from build123d import *

# Parameters (mm, degrees)
F0_W     = 35
F0_H     = 10.25
F0_W_2   = 10.25
F0_H_2   = 25
F1_DEPTH = 10
F2_R     = 10
F2_R_2   = 15
F3_DEPTH = 10


with BuildPart() as f1:
    # F0 (on Top) → F1 (new body)
    with BuildSketch(Plane.XY):
        with BuildLine():
            Line((140, 110), (-140, 110))
            ThreePointArc((-140, 110), (-147.071068, 107.071068), (-150, 100))
            Line((-150, 100), (-150, -100))
            ThreePointArc((-150, -100), (-147.071068, -107.071068), (-140, -110))
            Line((-140, -110), (140, -110))
            ThreePointArc((140, -110), (147.071068, -107.071068), (150, -100))
            Line((150, -100), (150, 100))
            ThreePointArc((150, 100), (147.071068, 107.071068), (140, 110))
        make_face()
        Polygon((-105.125, -100.125), (-140.125, -100.125), (-140.125, -75.125), (-129.875, -75.125), (-129.875, -89.878049), (-105.125, -89.875), align=None, mode=Mode.SUBTRACT)
        with Locations((-52.625, -95)):
            Rectangle(F0_W, F0_H, mode=Mode.SUBTRACT)
        with Locations((-135, -37.625)):
            Rectangle(F0_W_2, F0_H_2, mode=Mode.SUBTRACT)
        with Locations((52.625, -95)):
            Rectangle(F0_W, F0_H, mode=Mode.SUBTRACT)
        Polygon((129.875, -75.125), (140.125, -75.125), (140.125, -100.125), (105.125, -100.125), (105.125, -89.875), (129.875, -89.878049), align=None, mode=Mode.SUBTRACT)
        with Locations((135, -37.625)):
            Rectangle(F0_W_2, F0_H_2, mode=Mode.SUBTRACT)
        with Locations((-135, 37.625)):
            Rectangle(F0_W_2, F0_H_2, mode=Mode.SUBTRACT)
        Polygon((-129.875, 75.125), (-140.125, 75.125), (-140.125, 100.125), (-105.125, 100.125), (-105.125, 89.875), (-129.875, 89.878049), align=None, mode=Mode.SUBTRACT)
        with Locations((-52.625, 95)):
            Rectangle(F0_W, F0_H, mode=Mode.SUBTRACT)
        with Locations((135, 37.625)):
            Rectangle(F0_W_2, F0_H_2, mode=Mode.SUBTRACT)
        with Locations((52.625, 95)):
            Rectangle(F0_W, F0_H, mode=Mode.SUBTRACT)
        Polygon((105.125, 89.875), (105.125, 100.125), (140.125, 100.125), (140.125, 75.125), (129.875, 75.125), (129.875, 89.878049), align=None, mode=Mode.SUBTRACT)
    extrude(amount=F1_DEPTH)

    # F2 (on face) → F3 (cut)
    with BuildSketch(Plane.XY.offset(10)):
        with Locations((-83.84011, 16.042637)):
            Circle(F2_R)
        with Locations((-18.84011, 41.042637)):
            Circle(F2_R_2)
        with Locations((16.15989, 63.042637)):
            Circle(F2_R_2)
        with Locations((56.15989, 61.042637)):
            Circle(F2_R_2)
        with Locations((96.15989, 59.042637)):
            Circle(F2_R_2)
        with Locations((96.15989, 19.042637)):
            Circle(F2_R_2)
        with Locations((56.15989, 21.042637)):
            Circle(F2_R_2)
        with Locations((16.15989, 23.042637)):
            Circle(F2_R_2)
        with Locations((-18.84011, 1.042637)):
            Circle(F2_R_2)
    extrude(amount=-F3_DEPTH, mode=Mode.SUBTRACT)


solid = f1.part
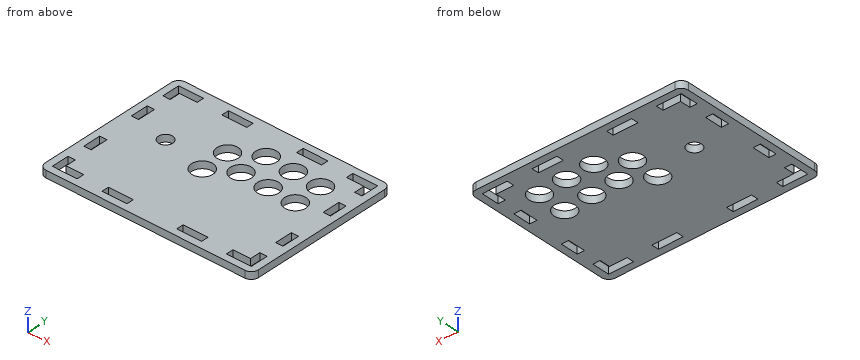
Geometry check sheet. Reference: the model listing, model coordinates, mm. Round coordinates to 2 decimals unless told otherwise and drop trailing zeros. Write each loop counter-clockwise with the first axis right and the second up, starting at its lowest first coordinate (ties: lowest second). Pieces come first, ordered by that corner, then holes.
Item 1: Go/stop test with a flat-tipped pin: pin 1 Ø5 at (x, y) = (-66, -64) entering from -Z. Record where the tip stops, or that it passes through.
Determined:
pin 1: stops at z = 0
Item 2: Section check D-D (x = 52). Record the boundary of the cut face in (y, z) (3 decimals).
Determined:
outline: (-110, 0) - (-100.125, 0) - (-100.125, 10) - (-110, 10) - close; (-89.875, 0) - (6.631, 0) - (6.631, 10) - (-89.875, 10) - close; (35.454, 0) - (46.631, 0) - (46.631, 10) - (35.454, 10) - close; (75.454, 0) - (89.875, 0) - (89.875, 10) - (75.454, 10) - close; (100.125, 0) - (110, 0) - (110, 10) - (100.125, 10) - close
Item 3: Material ranges on line 1 along Y through (x, z) = (112, 3.75) (3 decimals); line 2 along X through (y, z) = (-91, 9.75) (3 decimals); line 3 along X through (y, z) = (88.5, 4.25) (3 decimals), recorded low to high.
Determined:
line 1: y = -110 to -100.125, -89.876 to 89.876, 100.125 to 110
line 2: x = -150 to -140.125, -105.125 to -70.125, -35.125 to 35.125, 70.125 to 105.125, 140.125 to 150
line 3: x = -150 to -140.125, -129.875 to 129.875, 140.125 to 150
Item 4: Section check A-A (y = 81.5). Record the boundary of the cut face in (x, z) (3 decimals), plus the area to 4 significant figures.
Determined:
outline: (-150, 0) - (-140.125, 0) - (-140.125, 10) - (-150, 10) - close; (-129.875, 0) - (129.875, 0) - (129.875, 10) - (-129.875, 10) - close; (140.125, 0) - (150, 0) - (150, 10) - (140.125, 10) - close
area: 2,795 mm2
Item 5: Section check C-C (y = 30). Record the boundary of the cut face in (x, z) (3 decimals).
Determined:
outline: (-150, 0) - (-140.125, 0) - (-140.125, 10) - (-150, 10) - close; (-129.875, 0) - (-28.992, 0) - (-28.992, 10) - (-129.875, 10) - close; (-8.688, 0) - (2.871, 0) - (2.871, 10) - (-8.688, 10) - close; (29.449, 0) - (44.128, 0) - (44.128, 10) - (29.449, 10) - close; (68.192, 0) - (85.916, 0) - (85.916, 10) - (68.192, 10) - close; (106.404, 0) - (129.875, 0) - (129.875, 10) - (106.404, 10) - close; (140.125, 0) - (150, 0) - (150, 10) - (140.125, 10) - close
Item 6: Section check B-B (x = -63.5). Record the boundary of the cut face in (y, z) (3 decimals).
Determined:
outline: (-110, 0) - (-100.125, 0) - (-100.125, 10) - (-110, 10) - close; (-89.875, 0) - (89.875, 0) - (89.875, 10) - (-89.875, 10) - close; (100.125, 0) - (110, 0) - (110, 10) - (100.125, 10) - close
